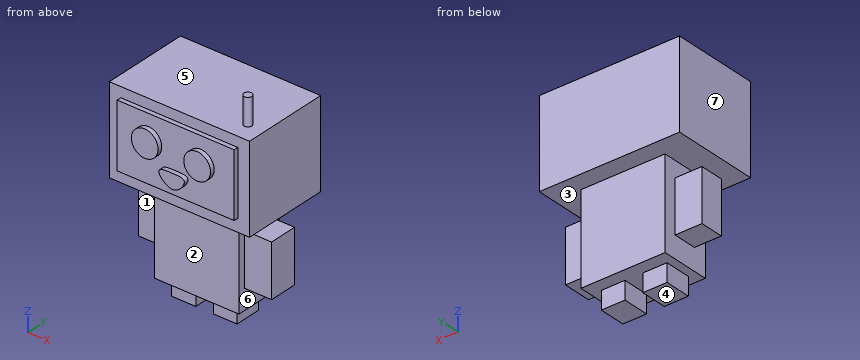
```python
from build123d import *

# Parameters (mm, degrees)
F0_W      = 39.7095009685
F0_H      = 24.7672665864
F1_DEPTH  = 24.765
F2_W      = 23.8453457132
F2_H      = 13.9918969944
F3_DEPTH  = 25.4
F4_W      = 6.7402645946
F4_H      = 14.7056742571
F5_DEPTH  = 7.62
F6_W      = 8.0039296299
F6_H      = 14.8659497499
F7_DEPTH  = 7.62
F8_W      = 6.8519285414
F8_H      = 7.4549559504
F8_W_2    = 6.698246114
F8_H_2    = 7.5303334743
F9_DEPTH  = 5.08
F10_W     = 33.1446304917
F10_H     = 18.2367824018
F11_DEPTH = 1.27
F12_R     = 3.790583573
F12_R_2   = 3.790584201
F13_DEPTH = 1.27
F14_R     = 1.1256242995
F15_DEPTH = 7.62


with BuildPart() as f1:
    # F0 (on Front) → F1 (new body)
    with BuildSketch(Plane.XZ):
        with Locations((-0.1829620451, 37.2313475236)):
            Rectangle(F0_W, F0_H)
    extrude(amount=F1_DEPTH)

    # F2 (on face) → F3 (join)
    with BuildSketch(Plane(origin=(0, 0, 24.8477142304), x_dir=(1, 0, 0), z_dir=(0, 0, -1))):
        with Locations((0.1507359557, 12.1197416447)):
            Rectangle(F2_W, F2_H)
    extrude(amount=F3_DEPTH)

    # F4 (on face) → F5 (join)
    with BuildSketch(Plane(origin=(-11.7719369009, 0, 0), x_dir=(0, -1, 0), z_dir=(-1, 0, 0))):
        with Locations((11.9688315317, 12.9703220446)):
            Rectangle(F4_W, F4_H)
    extrude(amount=F5_DEPTH)

    # F6 (on face) → F7 (join)
    with BuildSketch(Plane.YZ.offset(12.0734088123)):
        with Locations((-13.127992861, 12.5903561711)):
            Rectangle(F6_W, F6_H)
    extrude(amount=F7_DEPTH)

    # F8 (on face) → F9 (join)
    with BuildSketch(Plane(origin=(0, 0, -0.5522857696), x_dir=(1, 0, 0), z_dir=(0, 0, -1))):
        with Locations((-5.9734758688, 12.4474996701)):
            Rectangle(F8_W, F8_H)
        with Locations((5.8084283955, 12.4098109081)):
            Rectangle(F8_W_2, F8_H_2)
    extrude(amount=F9_DEPTH)

    # F10 (on face) → F11 (join)
    with BuildSketch(Plane.XZ.offset(24.765)):
        with Locations((-0.2155154943, 37.6151073724)):
            Rectangle(F10_W, F10_H)
    extrude(amount=F11_DEPTH)

    # F12 (on face) → F13 (join)
    with BuildSketch(Plane.XZ.offset(26.035)):
        with Locations((-7.9581402242, 39.5428165793)):
            Circle(F12_R)
        with Locations((6.8902717903, 39.42110762)):
            Circle(F12_R_2)
        with BuildLine():
            add(Edge.make_bspline(
                [(3.2390230335, 34.0659432113), (3.0810302353, 34.9220679818), (0.036704506, 34.8800177819), (-6.049244101, 35.0644989514), (0.143997862, 28.5163578143), (3.4244660087, 33.0610725698), (3.2390230335, 34.0659432113)],
                knots=[0, 0, 0, 0, 0.2217830764, 0.4651495707, 0.7396836186, 1, 1, 1, 1], degree=3))
        make_face()
    extrude(amount=F13_DEPTH)

    # F14 (on face) → F15 (join)
    with BuildSketch(Plane.XY.offset(49.6149808168)):
        with Locations((14.9038648233, -19.4570012391)):
            Circle(F14_R)
    extrude(amount=F15_DEPTH)


solid = f1.part
```
Geometry check sheet. Reference: the model listing, model coordinates, mm. Face numbers are marked on the shaded views. A direction names the side the tool comes from. Coordinates: 2 decimals unless noted, no trailing zeros. Write each loop counter-clockwise with the first axis right and the second up, starting at its lowest first coordinate (ties: lowest second). Pieces come first, ordered by that corner, then holes. Notation, with made-up numbers: M 5,75.25 L 16,75.25 A25 cw 16,107.25 Z; hole C 1,-38.5 d6. An arc over 180 degrees is marked long. Answer as a JSON object with one key per item and string values.
1. Tool access check on the marked faces 1, 2 and 3. Record the directions out of +Z, -Z, +X, -X, +Y, -Y that give a thin tool (end or side, any length) a straight path to the whole face; none if there is none.
Answers below:
{"face 1": "-Z, -X, -Y", "face 2": "-Z, +X, -X, -Y", "face 3": "none"}
2. Section check B-B, the plane y = -11. Enter the section's corners in (x, z).
Answers below:
{"outline": "M -20.04,24.85 L -11.77,24.85 L -11.77,20.32 L -19.39,20.32 L -19.39,5.62 L -11.77,5.62 L -11.77,-0.55 L -9.4,-0.55 L -9.4,-5.63 L -2.55,-5.63 L -2.55,-0.55 L 2.46,-0.55 L 2.46,-5.63 L 9.16,-5.63 L 9.16,-0.55 L 12.07,-0.55 L 12.07,5.16 L 19.69,5.16 L 19.69,20.02 L 12.07,20.02 L 12.07,24.85 L 19.67,24.85 L 19.67,49.61 L -20.04,49.61 Z"}
3. Scan lines: L1, parallel to X at y = -11.25, z = -3; L2, parallel to Z at x = 13, y = -12; L3, parallel to Z at x = -4.5, y = -12.75. Record each from-to range of solid material in increasing order.
Answers below:
{"L1": "x = -9.4 to -2.55, 2.46 to 9.16", "L2": "z = 5.16 to 20.02, 24.85 to 49.61", "L3": "z = -5.63 to 49.61"}
4. Section check D-D, the plane z = 8. Enter the section's corners in (x, y).
Answers below:
{"outline": "M -19.39,-15.34 L -11.77,-15.34 L -11.77,-19.12 L 12.07,-19.12 L 12.07,-17.13 L 19.69,-17.13 L 19.69,-9.13 L 12.07,-9.13 L 12.07,-5.12 L -11.77,-5.12 L -11.77,-8.6 L -19.39,-8.6 Z"}
5. Go/stop test with flat-tipped pins: pin 1 Ø10 at (y, z) = (-6, 31.5) entering from +X; pin 2 Ø1 at (y, z) = (-25.5, 42) entering from -X; pin 3 Ø8.5 at (x, z) = (17.5, 11.5) entering from -Y. Record where each tip stops, or that it passes through.
Answers below:
{"pin 1": "stops at x = 19.67", "pin 2": "stops at x = -16.79", "pin 3": "stops at y = -17.13"}
6. Section check A-A, the plane z = -1.5. Enter the section's corners in (x, y), plus the area to 3 significant figures.
Answers below:
{"outline": "M -9.4,-16.17 L -2.55,-16.17 L -2.55,-8.72 L -9.4,-8.72 Z; M 2.46,-16.17 L 9.16,-16.17 L 9.16,-8.64 L 2.46,-8.64 Z", "area": "102 mm²"}
7. Section check C-C, the plane x = 4.5. Enter the section's corners in (y, z) (1 decimal).
Answers below:
{"outline": "M -27.3,36.5 L -26,36.5 L -26,28.5 L -24.8,28.5 L -24.8,24.8 L -19.1,24.8 L -19.1,-0.6 L -16.2,-0.6 L -16.2,-5.6 L -8.6,-5.6 L -8.6,-0.6 L -5.1,-0.6 L -5.1,24.8 L 0,24.8 L 0,49.6 L -24.8,49.6 L -24.8,46.7 L -26,46.7 L -26,42.4 L -27.3,42.4 Z"}
8. Draft check along Z on the marked faces 4, 5, 6 and 7. Enter one of: released by +Z, released by -Z, zero draft, split by the parting line, or undercut.
Answers below:
{"face 4": "released by -Z", "face 5": "released by +Z", "face 6": "undercut", "face 7": "zero draft"}
